Source: three-view drawing plus pictorial views. Frame: mm from the lowest corner of the part. Coordinates: 2 decimals unless noted, no trailing zeros. Loops run counter-clockwise (first coordinate to the right, second up) from the corner with the lowest first, then second, coordinate; pieces in that order, holes last.
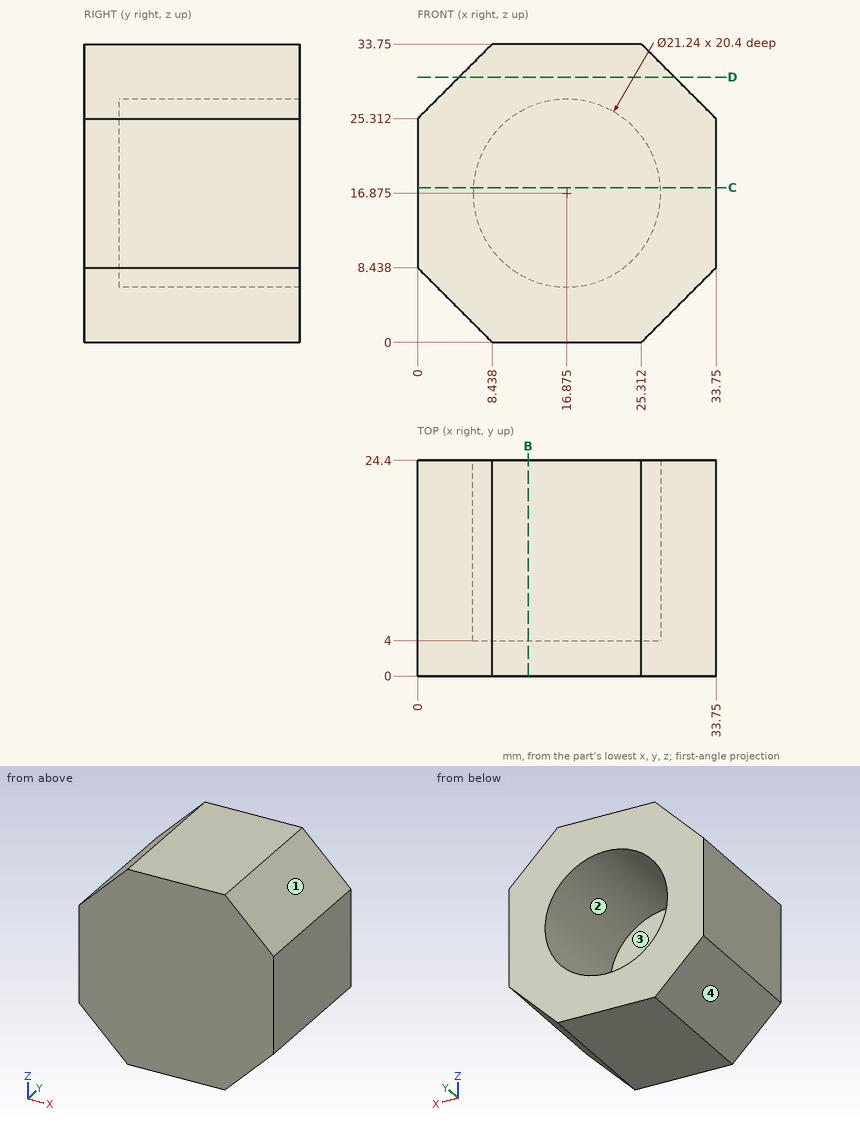
Q1. Section D-D, the plane z = 30. Return the cut outline in (x, y).
Q2. Section B-B, the plane x = 12.5. Return the cut outline in (y, z).
Q3. Contact query for a flat-ended pin moving along its axis: pin 1 Ø17 at (x, z) = (18.5, 16.5) entering from +Y. Output: stop coordinate, or through.
Q4. Draft query along X for the marked faces 1, 2, 3 and 4. Return one class per face: +X half, -X half, draft (parallel to the pull), parting line (faces both ways), or undercut.
Q5. Section C-C, the plane z = 17.5. Return the cut outline in (x, y), plus the area to 3 significant figures.
Q6. Line query: line 1 along Y through (x, z) = (19.5, 22); line 2 along Z through (x, y) = (17.5, 15.75); line 3 along X through (y, z) = (22, 13). Output: solid intervals per line, ascending.
Derived:
1. outline: (4.69, 0) - (29.06, 0) - (29.06, 24.4) - (4.69, 24.4) - close
2. outline: (0, 0) - (24.4, 0) - (24.4, 7.2) - (4, 7.2) - (4, 26.55) - (24.4, 26.55) - (24.4, 33.75) - (0, 33.75) - close
3. pin 1: stops at y = 4
4. face 1: +X half
4. face 2: undercut
4. face 3: undercut
4. face 4: -X half
5. outline: (0, 0) - (33.75, 0) - (33.75, 24.4) - (27.48, 24.4) - (27.48, 4) - (6.27, 4) - (6.27, 24.4) - (0, 24.4) - close
5. area: 391 mm2
6. line 1: y = 0 to 4
6. line 2: z = 0 to 6.27, 27.48 to 33.75
6. line 3: x = 0 to 6.99, 26.76 to 33.75
